Geometry: see drawing. Coordinates: mm, zero at the bounding-box minimum. A direction names the side the tool comes from. Give positions to 0.01 mm unless a question says otherwise; leave off trailing zeros. Order: outer loops, then holes, each group sorted by start corner. A loop starts at its lowest first (then second) coordinate and runs counter-clockwise, first axis right, second up. Notation, with made-up numbers: M -38.75,5.25 L -11.75,5.25 A19 cw -11.75,29.25 Z; hole C 61.25,1 d9. An arc over 180 degrees is marked long. Answer as a JSON object with one key per item and string values. Group by question number.
1. Pin query (flat end, axial travel): P1, Ø3, axis at x = 5, y = 22.5, coming from the -Z side; P2, Ø3, axis at x = 7, y = 31.5, coming from the -Z side. Return the tip coordinate at first contact, or that it passes through.
2. Section query D-D (x = 8). Output: boundary loops of the cut face in (y, z).
3. Section query C-C (z = 1.4). Output: boundary loops of the cut face in (x, y).
4. Material intervals for L1, parallel to X at y = 22.5, z = 2.2; L2, parallel to Z at x = 5, y = 5; L3, parallel to Y at x = 5, z = 4.5, sorted ascending. Write a range as [from, to].
5. Section query A-A (y = 22.5). Output: boundary loops of the cut face in (x, z), plus the area to 3 significant figures.
6. Section query B-B (x = 5). Output: boundary loops of the cut face in (y, z), plus the area to 3 significant figures.
7. Set-up query: the marked faces 1 and 2. Return all of +Z, -Z, +X, -X, +Y, -Y with unobstructed straight access to the full face (end or side cutting, diameter ignored); none if empty.
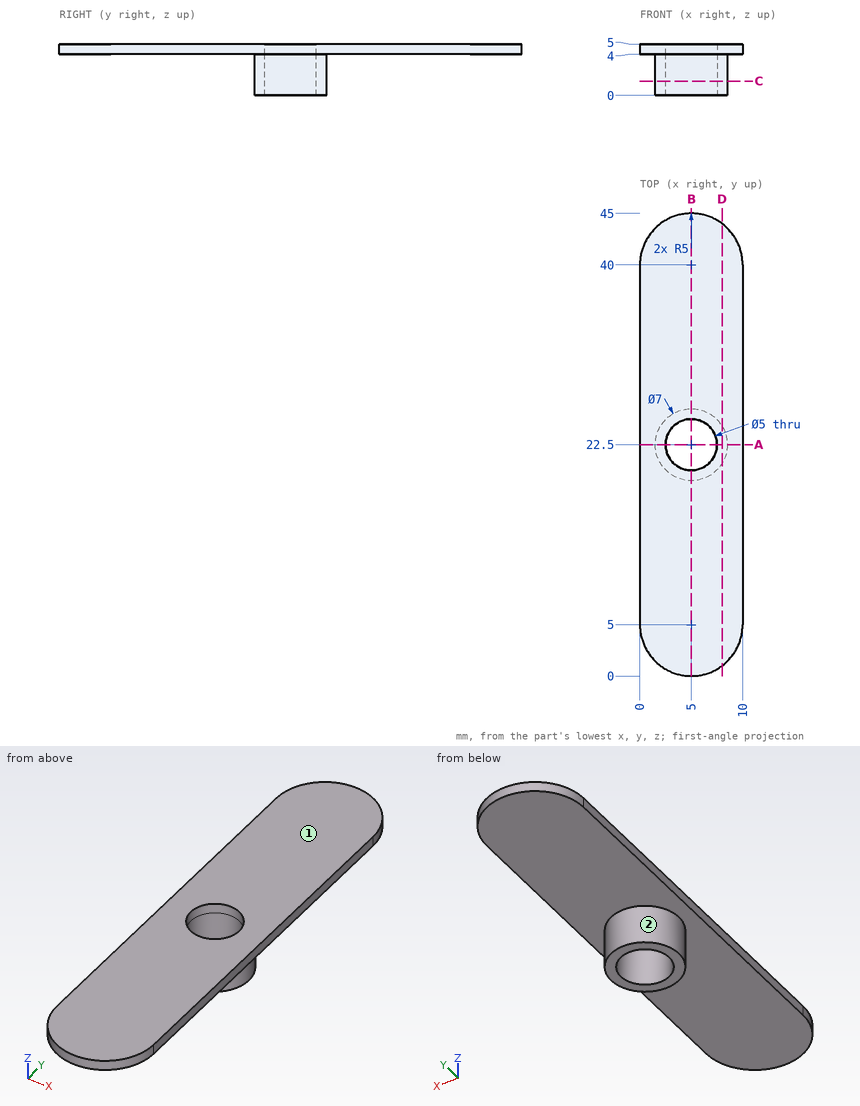
Answer sheet:
{
 "1": {"P1": "through", "P2": "z = 4"},
 "2": {"outline": "M 1,4 L 20.7,4 L 20.7,0 L 24.3,0 L 24.3,4 L 44,4 L 44,5 L 1,5 Z"},
 "3": {"outline": "C 5,22.5 d7; hole C 5,22.5 d5"},
 "4": {"L1": "[1.5, 2.5], [7.5, 8.5]", "L2": "[4, 5]", "L3": "[0, 20], [25, 45]"},
 "5": {"outline": "M 0,4 L 1.5,4 L 1.5,0 L 2.5,0 L 2.5,5 L 0,5 Z; M 7.5,0 L 8.5,0 L 8.5,4 L 10,4 L 10,5 L 7.5,5 Z", "area": "13.0 mm^2"},
 "6": {"outline": "M 0,4 L 19,4 L 19,0 L 20,0 L 20,5 L 0,5 Z; M 25,0 L 26,0 L 26,4 L 45,4 L 45,5 L 25,5 Z", "area": "48.0 mm^2"},
 "7": {"face 1": "+Z, +X, -X, +Y, -Y", "face 2": "-Z"}
}
